Can you work these out from the drawing? Everything is in mm from the part's minimum corner. A direction names the side the tool comes from. Coordinates: 2 decimals unless noted, no trailing zeros. Order: outer loops, then holes, each group sorted by start corner. A loop starts at its lowest first (then second) coordinate and runs counter-clockwise, first axis right, second up. Notation, with made-up numbers: M 2.5,-7 L 17.5,-7 A18 cw 17.5,19 Z; hole C 33,-9 d6. An arc over 180 degrees is marked long. Answer as a JSON object with one key per item and string values.
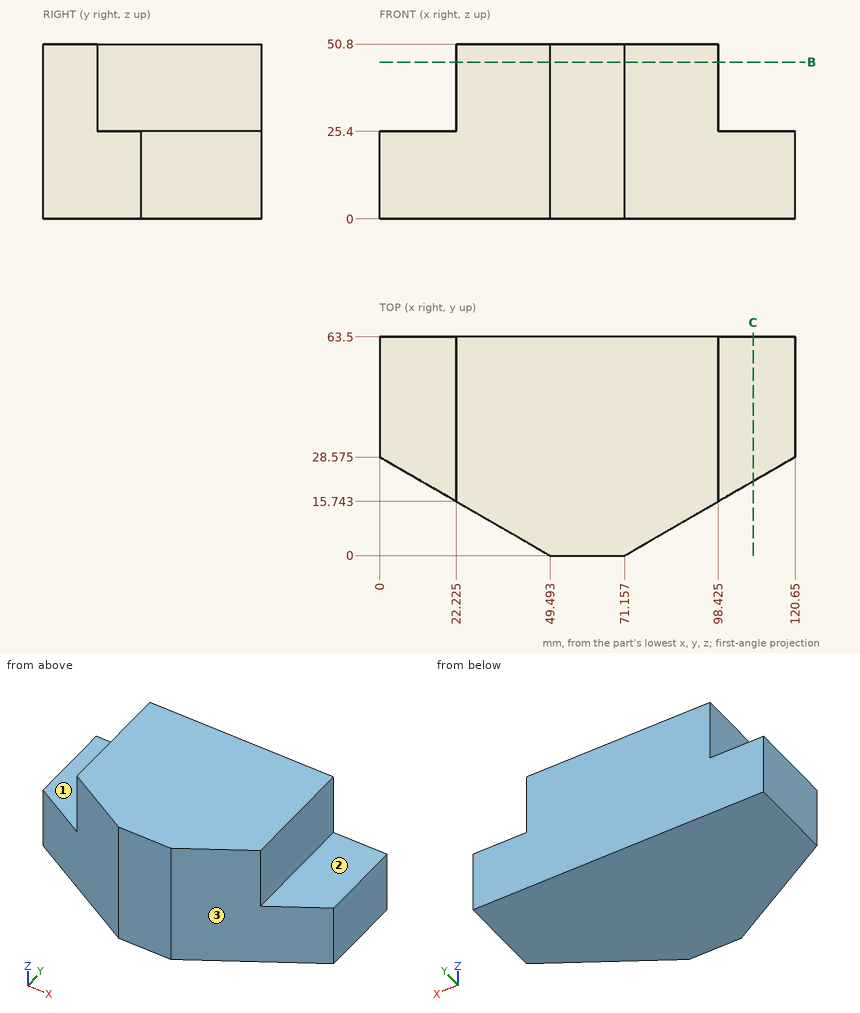
Item 1: Please list where these lines run through material, in increasing order: line 1 (Z direction, x = 11, y = 53); line 2 (X direction, y = 36, z = 47.5) (1 decimal); line 3 (Y direction, x = 27, z = 24.5) (1 decimal).
Answers follow:
{"line 1": "z = 0 to 25.4", "line 2": "x = 22.2 to 98.4", "line 3": "y = 13 to 63.5"}
Item 2: I'm going to push flat-ended pins straight in: pin 1 (12.5 mm diameter, centred on y = 30.5, z = 42.5, fed in from -X) (3 decimals); pin 2 (2 mm diameter, centred on x = 20.5, z = 38, fed in from -Y); pin 3 (10 mm diameter, centred on y = 20.5, z = 45.5, fed in from +X) (3 decimals); pin 4 (6.5 mm diameter, centred on x = 10, y = 39.5, fed in from +Z). Where does each tip first touch, or does it pass through?
Answers follow:
{"pin 1": "stops at x = 22.225", "pin 2": "passes through", "pin 3": "stops at x = 98.425", "pin 4": "stops at z = 25.4"}
Item 3: I want a section at C-C, the plane x = 108.5. Write out the boundary of the cut face in (y, z), plus the area to 3 significant figures.
Answers follow:
{"outline": "M 21.56,0 L 63.5,0 L 63.5,25.4 L 21.56,25.4 Z", "area": "1,070 mm^2"}
Item 4: I want a section at B-B, the plane z = 45.5. Write out the boundary of the cut face in (x, y) (1 decimal).
Answers follow:
{"outline": "M 22.2,15.7 L 49.5,0 L 71.2,0 L 98.4,15.7 L 98.4,63.5 L 22.2,63.5 Z"}
Item 5: Which directions (+Z, -Z, +X, -X, +Y, -Y) give clear straight access to the entire face, cutting with the end or side of a thin tool? Please do the marked faces 1, 2 and 3.
Answers follow:
{"face 1": "+Z, -X, +Y, -Y", "face 2": "+Z, +X, +Y, -Y", "face 3": "+Z, -Z, +X, -Y"}
